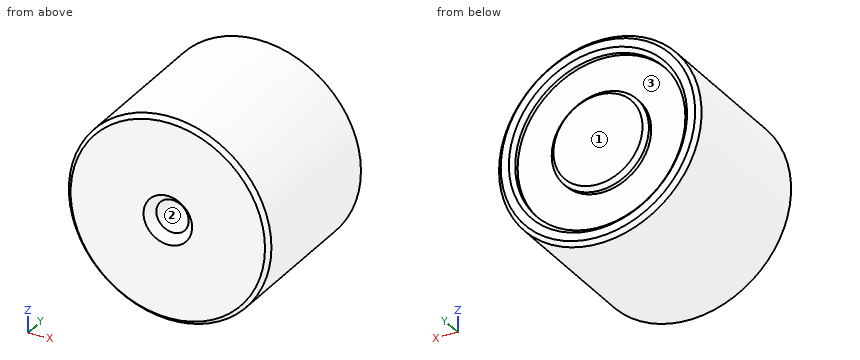
from build123d import *

# Parameters (mm, degrees)
SKETCH_1_R          = 12.5
EXTRUDE_1_DEPTH     = 20
SKETCH_2_R          = 10.5
SKETCH_2_R_2        = 6
CUT_EXTRUDE_1_DEPTH = 1
CHAMFER_1_SIZE      = 0.5
SKETCH_3_R          = 2
CUT_EXTRUDE_2_DEPTH = 12
CHAMFER_2_SIZE      = 1


with BuildPart() as part:
    # Эскиз1 → Бобышка-Вытянуть1 (new body)
    with BuildSketch(Plane(origin=(0, 0, 0), x_dir=(1, 0, 0), z_dir=(0, 1, 0))):
        Circle(SKETCH_1_R)
    extrude(amount=EXTRUDE_1_DEPTH)

    # Эскиз2 → Вырез-Вытянуть1 (cut)
    with BuildSketch(Plane(origin=(0, 20, 0), x_dir=(1, 0, 0), z_dir=(0, 1, 0))):
        Circle(SKETCH_2_R)
        Circle(SKETCH_2_R_2, mode=Mode.SUBTRACT)
    extrude(amount=-CUT_EXTRUDE_1_DEPTH, mode=Mode.SUBTRACT)

    # Фаска1
    chamfer_1_edges = [part.edges().sort_by_distance(p)[0] for p in [
        (-12.5, 0, 0),
        (-12.5, 20, 0),
        (-10.5, 20, 0),
        (-6, 20, 0),
    ]]
    chamfer(chamfer_1_edges, length=CHAMFER_1_SIZE)

    # Эскиз3 → Вырез-Вытянуть2 (cut)
    with BuildSketch(Plane.XZ):
        Circle(SKETCH_3_R)
    extrude(amount=-CUT_EXTRUDE_2_DEPTH, mode=Mode.SUBTRACT)

    # Фаска2
    chamfer_2_edges = [part.edges().sort_by_distance(p)[0] for p in [
        (-2, 0, 0),
    ]]
    chamfer(chamfer_2_edges, length=CHAMFER_2_SIZE)


solid = part.part
Verification items for the finished model (mm, model axes). Face numbers are marked on the shaded views. A direction names the side the tool comes from. Coordinates: 2 decimals unless noted, no trailing zeros. Write each loop counter-clockwise with the first axis right and the second up, starting at its lowest first coordinate (ties: lowest second). Pieces come first, ordered by that corner, then holes. Notation, with made-up numbers: M -36,61.25 L -14,61.25 A21 ccw -14,77.25 Z; hole C 54.25,27 d3. An arc over 180 degrees is marked long. Use CSV: the item, a comma, the result in double quotes.
Q1. Set-up check for the marked faces 1, 2 and 3: record each of +Z, -Z, +X, -X, +Y, -Y from which the full face is reachable in a straight line by a thin tool's end or side.
Computed values:
face 1,"+Z, -Z, +X, -X, +Y"
face 2,"-Y"
face 3,"+Y"
Q2. Section check C-C, the plane y = 2. Enter the section's corners in (x, z), and give its area (3 significant figures).
Computed values:
outline,"C 0,0 d25; hole C 0,0 d4"
area,"478 mm²"
Q3. Section check B-B, the plane x = 0. Enter the section's corners in (y, z).
Computed values:
outline,"M 0,-12 L 0.5,-12.5 L 19.5,-12.5 L 20,-12 L 20,-11 L 19.5,-10.5 L 19,-10.5 L 19,-6 L 19.5,-6 L 20,-5.5 L 20,5.5 L 19.5,6 L 19,6 L 19,10.5 L 19.5,10.5 L 20,11 L 20,12 L 19.5,12.5 L 0.5,12.5 L 0,12 L 0,3 L 1,2 L 12,2 L 12,-2 L 1,-2 L 0,-3 Z"
Q4. Go/stop test with flat-tipped pins: P1, Ø1.5, axis at x = -4.5, z = 0, coming from the -Y side; P2, Ø2, axis at x = 9.5, y = 5.5, coming from the -Z side; P3, Ø1.2, axis at x = 1, z = -0.5, coming from the -Y side; P4, Ø4, axis at x = 7.5, y = 11.5, coming from the +Z side (3 decimals). Record where each tip stops, or that it passes through.
Computed values:
P1,"y = 0"
P2,"z = -9.17"
P3,"y = 12"
P4,"z = 11.225"
Q5. Thickness scan on line 1 along Z through (x, y) = (0, 19.2); line 2 along Z through (x, y) = (0, 4.5); line 3 along Y through (x, z) = (-7.75, 5.5). Record the ranges inside material, lowest first. Write a range as [from, to].
Computed values:
line 1,"[-12.5, -10.5], [-6, 6], [10.5, 12.5]"
line 2,"[-12.5, -2], [2, 12.5]"
line 3,"[0, 19]"
Q6. Section check A-A, the plane z = 0. Enter the section's corners in (x, y).
Computed values:
outline,"M -12.5,0.5 L -12,0 L -3,0 L -2,1 L -2,12 L 2,12 L 2,1 L 3,0 L 12,0 L 12.5,0.5 L 12.5,19.5 L 12,20 L 11,20 L 10.5,19.5 L 10.5,19 L 6,19 L 6,19.5 L 5.5,20 L -5.5,20 L -6,19.5 L -6,19 L -10.5,19 L -10.5,19.5 L -11,20 L -12,20 L -12.5,19.5 Z"
